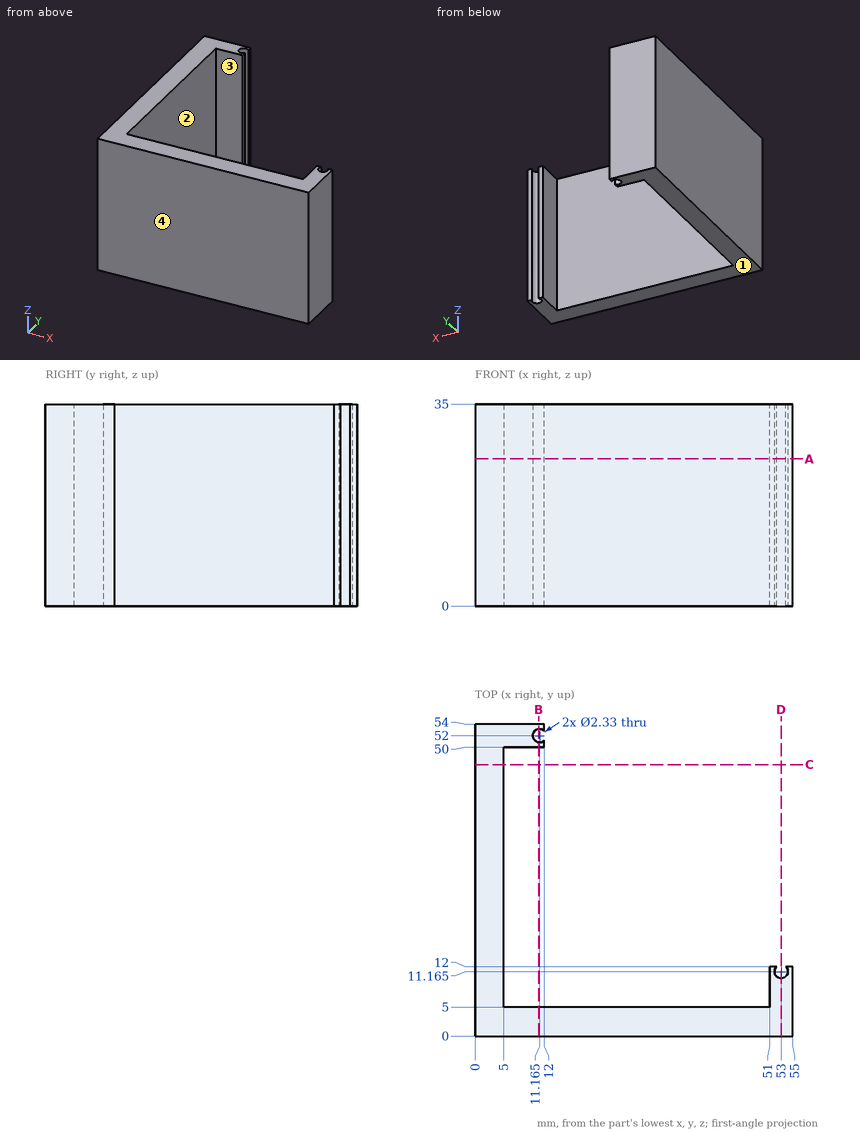
The drawing under review shows one solid part. Ordinate dimensions are in mm from its lowest x, y, z. Give positions to 0.01 mm unless a question says otherwise; leave off trailing zeros. Loops run counter-clockwise (first coordinate to the right, second up) from the corner with the lowest first, then second, coordinate; pieces in that order, holes last. Notation, with made-up numbers: M -7,86.25 L 20,86.25 A29 ccw 20,110.25 Z; hole C -29.5,-35 d11. An arc over 180 degrees is marked long. One line per question, with ' | ' between items. Start each with the question number.
1. Insertion check: P1, Ø5, axis at y = 47.5, z = 27.5, coming from the -X side; P2, Ø1.3, axis at x = 51.5, z = 23.5, coming from the +Y side; P3, Ø2, axis at x = 7.5, y = 40, coming from the -Z side; P4, Ø0.6, axis at y = 53.5, z = 21.5, coming from the +X side. Each pin has a flat end and moves straight along its axis. Give the tip position at first contact, or say it passes through.
2. Add section B-B (x = 11). Write out the cut boundary in (y, z).
3. To check wall thickness, follow L1, parallel to X at y = 5.5, z = 15; L2, parallel to Y at x = 10.5, z = 33.5; L3, parallel to X at y = 52, z = 17. State the ranges of each line that lie inside material, in increasing order.
4. The part is to be moulded in two halves that separate along Y. For the marked faces 1, 2, 3 and 4, say which applies: released by +Y, released by -Y, zero draft, split by the parting line, or undercut.
5. Add section A-A (z = 25.5). Write out the cut boundary in (x, y) (3 decimals).
6. Add section D-D (x = 53). Write out the cut boundary in (y, z).
7. Add section C-C (y = 47). Write out the cut boundary in (x, z), plus the area to 3 significant figures.
Worked out:
1) P1: stops at x = 0 | P2: stops at y = 12 | P3: passes through | P4: stops at x = 12
2) outline: M 0,0 L 5,0 L 5,35 L 0,35 Z; M 50,0 L 50.85,0 L 50.85,35 L 50,35 Z; M 53.15,0 L 54,0 L 54,35 L 53.15,35 Z
3) L1: x = 0 to 5, 51 to 55 | L2: y = 0 to 5, 50 to 51.04, 52.96 to 54 | L3: x = 0 to 10
4) face 1: zero draft | face 2: undercut | face 3: undercut | face 4: released by -Y
5) outline: M 0,0 L 55,0 L 55,12 L 53.812,12 A1.165 cw long 52.188,12 L 51,12 L 51,5 L 5,5 L 5,50 L 12,50 L 12,51.188 A1.165 cw long 12,52.812 L 12,54 L 0,54 Z
6) outline: M 0,0 L 10,0 L 10,35 L 0,35 Z
7) outline: M 0,0 L 5,0 L 5,35 L 0,35 Z | area: 175 mm²
